Design review of the part shown in the three views and the two pictorial views. Dimensions are in mm from the part's minimum x, y and z. A direction names the side the tool comes from. Round coordinates to 2 decimals unless told otherwise and drop trailing zeros. Loops run counter-clockwise (first coordinate to the right, second up) from the corner with the lowest first, then second, coordinate; pieces in that order, holes last. Notation, with made-up numbers: M 1.5,-30.5 L 32.5,-30.5 A20 cw 32.5,-14.5 Z; hole C 65.5,82 d3. An arc over 180 degrees is marked long. One line per question, with ' | ' between items. Start each with the question number.
1) For pin 1 Ø5 at (x, y) = (2.5, 3.5) entering from -Z, flat-tipped, find the tip position at first contact; note if it passes through.
2) We need section D-D (x = 4.25). Give the boundary of the cut face in (y, z).
3) We need section A-A (y = 6). Give the boundary of the cut face in (x, z) (1 decimal).
4) We need section C-C (y = 1.25). Give the boundary of the cut face in (x, z) (1 decimal), and give its area (3 significant figures).
5) For the marked faces 1 and 2, list the 3-axis set-ups (+Z, -Z, +X, -X, +Y, -Y) from which the entire face can be reached by the end or side of a thin tool; tool diameter is ignored.
6) We need section B-B (z = 9.5). Give the boundary of the cut face in (x, y) (1 decimal).
7) Mouldability with a two-part tool opening along X and no side actions: class the marked faces 3, 4, 5 and 6 as pulls with the +X half, pulls with the -X half, needs draft (parallel to the pull), parting line crosses it, or undercut.
8) For probe 1 along Y at (x, z) = (8.3, 3.5) (1 decimal); probe 2 along Y at (x, z) = (2.5, 5); probe 3 along X at (y, z) = (3.75, 9.75) (1 decimal), list the stretches that pass through material, from the lowest coordinate up. Write a range as from..to.
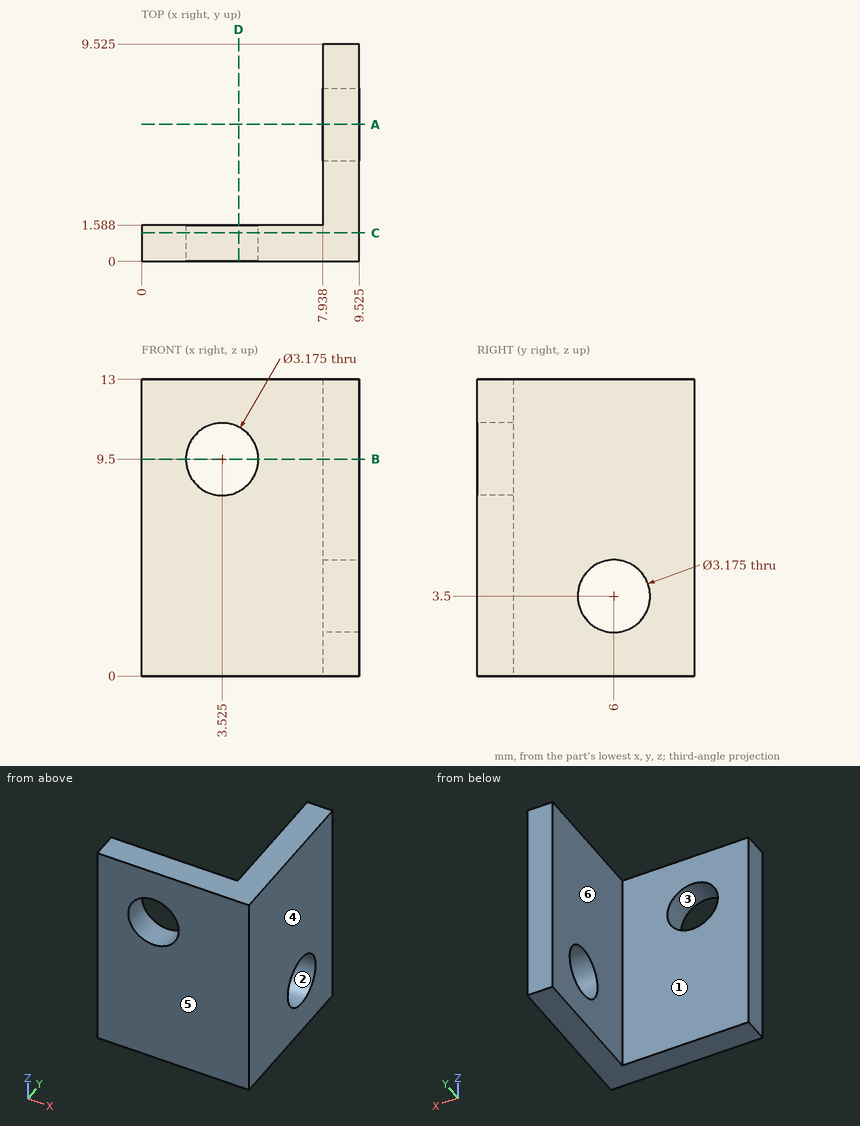
Answers below:
1) pin 1: z = 0
2) outline: M 0,0 L 1.59,0 L 1.59,8.09 L 0,8.09 Z; M 0,10.91 L 1.59,10.91 L 1.59,13 L 0,13 Z
3) outline: M 7.9,0 L 9.5,0 L 9.5,1.9 L 7.9,1.9 Z; M 7.9,5.1 L 9.5,5.1 L 9.5,13 L 7.9,13 Z
4) outline: M 0,0 L 9.5,0 L 9.5,13 L 0,13 Z; hole C 3.5,9.5 d3.2 | area: 116 mm^2
5) face 1: +Z, -Z, -X, +Y | face 2: +X, -X
6) outline: M 0,0 L 1.9,0 L 1.9,1.6 L 0,1.6 Z; M 5.1,0 L 9.5,0 L 9.5,9.5 L 7.9,9.5 L 7.9,1.6 L 5.1,1.6 Z
7) face 3: undercut | face 4: pulls with the +X half | face 5: needs draft | face 6: pulls with the -X half
8) probe 1: 0..4.4, 7.6..9.5 | probe 2: 0..1.59 | probe 3: 7.9..9.5
